```python
from build123d import *

# Parameters (mm, degrees)
ENL_V_MAT_EXTRU_6_DEPTH = 25


with BuildPart() as part:
    # Esquisse1 → Révolution1 (revolve)
    with BuildSketch(Plane.XY):
        with BuildLine():
            Line((0, 0), (-120, 0))
            Line((-120, 0), (-120, 7.5))
            ThreePointArc((-120, 7.5), (-119.707106781, 8.207106781), (-119, 8.5))
            Line((-119, 8.5), (-90, 8.5))
            Line((-90, 8.5), (-90, 10.5))
            ThreePointArc((-90, 10.5), (-89.707106781, 11.207106781), (-89, 11.5))
            Line((-89, 11.5), (-41, 11.5))
            ThreePointArc((-41, 11.5), (-40.292893219, 11.207106781), (-40, 10.5))
            Line((-40, 10.5), (-40, 8.5))
            Line((-40, 8.5), (0, 8.5))
            Line((0, 8.5), (0, 0))
        make_face()
    revolve(axis=Axis((0, 0, 0), (-1, 0, 0)))

    # Esquisse6 → Enlèv. mat.-Extru.6 (cut)
    with BuildSketch(Plane(origin=(0, 0, 0), x_dir=(0, 0, -1), z_dir=(1, 0, 0))):
        Polygon((-6.5, 9.404987847), (-6.5, -10.595012153), (-12.325260954, -10.595012153), (-12.325260954, 19.404987847), (-6.5, 19.404987847), align=None)
    extrude(amount=-ENL_V_MAT_EXTRU_6_DEPTH, mode=Mode.SUBTRACT)


solid = part.part
```
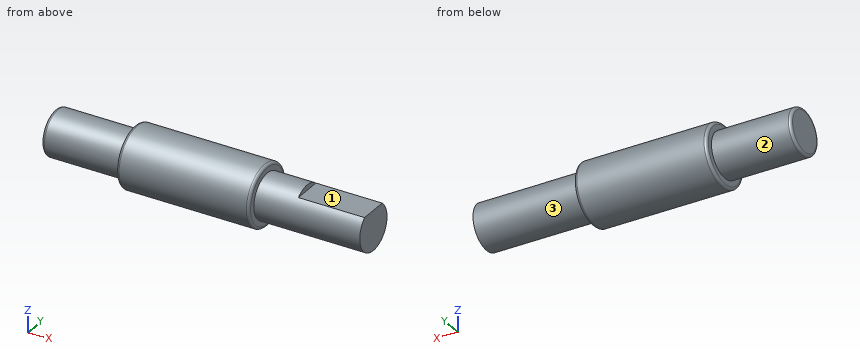
Work out the finished part from the listing and answer in its coordinate system (mm). Face numbers are marked on the shaded views. A direction names the side the tool comes from. Round coordinates to 2 decimals unless told otherwise and drop trailing zeros. Order: outer loops, then holes, each group sorted by start corner. A loop starts at its lowest first (then second) coordinate and runs counter-clockwise, first axis right, second up.
Q1. A cutting plane is placed at B-B, the plane z = 0. Determine the outline of the cut face in (x, y), then the cut area to 3 significant figures.
Solution:
outline: (-120, -7.5) arc R1 ccw to (-119, -8.5) - (-90, -8.5) - (-90, -10.5) arc R1 ccw to (-89, -11.5) - (-41, -11.5) arc R1 ccw to (-40, -10.5) - (-40, -8.5) - (0, -8.5) - (0, 8.5) - (-40, 8.5) - (-40, 10.5) arc R1 ccw to (-41, 11.5) - (-89, 11.5) arc R1 ccw to (-90, 10.5) - (-90, 8.5) - (-119, 8.5) arc R1 ccw to (-120, 7.5) - close
area: 2,340 mm2
Q2. A cutting plane is placed at C-C, the plane x = -51. Determine the outline of the cut face in (y, z).
Solution:
outline: circle Ø23 at (0, 0)
Q3. A cutting plane is placed at D-D, the plane x = -91. Determine the outline of the cut face in (y, z).
Solution:
outline: circle Ø17 at (0, 0)
Q4. A cutting plane is placed at A-A, the plane y = 0. Determine the outline of the cut face in (x, z).
Solution:
outline: (-120, -7.5) arc R1 ccw to (-119, -8.5) - (-90, -8.5) - (-90, -10.5) arc R1 ccw to (-89, -11.5) - (-41, -11.5) arc R1 ccw to (-40, -10.5) - (-40, -8.5) - (0, -8.5) - (0, 6.5) - (-25, 6.5) - (-25, 8.5) - (-40, 8.5) - (-40, 10.5) arc R1 ccw to (-41, 11.5) - (-89, 11.5) arc R1 ccw to (-90, 10.5) - (-90, 8.5) - (-119, 8.5) arc R1 ccw to (-120, 7.5) - close
Q5. A tool of negligible diameter and unlimited length cuts with its end or side. For the marked faces 1, 2 and 3, from which of +Z, -Z, +X, -X, +Y, -Y can it reach the whole face along a straight path? Write none if from no direction.
Solution:
face 1: +Z, +X, +Y, -Y
face 2: -X
face 3: +X
Q6. Find the intervals of material crossed by line 1 along Y through (x, z) = (-82, -0.75); line 2 along X through (y, z) = (8, 6); line 3 along Y through (x, z) = (-8.5, -6.5), in increasing order.
Solution:
line 1: y = -11.48 to 11.48
line 2: x = -90 to -40
line 3: y = -5.48 to 5.48
Q7. Given pin 1 Ø1 at (x, z) = (-28, -7) entering from +Y; pin 2 Ø2 at (x, z) = (-17, -2.5) entering from -Y; pin 3 Ø3.5 at (x, y) = (-15, 1.5) entering from +Z, each flat-ended and moving along its own axis, determine where each tip first touches the part or whether it passes through.
Solution:
pin 1: stops at y = 5.48
pin 2: stops at y = -8.37
pin 3: stops at z = 6.5
